Read the model definition and answer for the solid it produces. Units are mm, in the model's axes. A direction names the side the tool comes from. Coordinates: 2 decimals unless noted, no trailing zeros. Loops run counter-clockwise (first coordinate to the right, second up) from the corner with the lowest first, then second, coordinate; pieces in that order, holes last. Notation, with made-up numbers: M 80,82 L 131,82 A25 ccw 131,107 Z; hole C 24,-34 d4. An arc over 180 degrees is marked long. One line per item, written item: value. Start each with the question number.
1. Consider probe 1 along Y at (x, z) = (0, 4.15); probe 2 along X at (y, z) = (-7, 1.5); probe 3 along Y at (x, z) = (-2, -1.5). Determine where each line is inside the solid, lowest interval first.
2. For faces 4 (the face through (9, 6, 1.118)), 5 (the face through (-3.26, -14.68, -1.39)), 6 (the face through (10, -10, -2.134)), 7 (the face through (-3, -8, 3.734)), determine the directions among +Z, -Z, +X, -X, +Y, -Y from which every point of the face is accessible in a straight line to the end or side of a thin tool.
3. Determine the mould class of faces 1 (the face through (10, -10, 2.134)), 2 (the face through (8.89, 2.8, -3.29)), 3 (the face through (-8.03, 0.35, 4.07)) for opening direction X: +X half, -X half, draft (parallel to the pull), parting line (faces both ways), or undercut.
4. Flat-ended cylindrical pins translate along their axes: pin 1 (10.5 mm diameter, centred on x = 0, y = 0, fed in from -Z); pin 2 (1.5 mm diameter, centred on y = 10.5, z = 0.5, fed in from +X); pin 3 (2 mm diameter, centred on x = 0, y = -12, fed in from +Z); pin 4 (1.5 mm diameter, centred on x = 2, z = -0.5, fed in from -Y). Find the tip coordinate at first contact, or state that the pin passes through.
5. The part is cut by section A-A (z = -3.25). Write down the section's boundary in (x, y), then the cut area to 3 significant figures.
```python
from build123d import *
from build123d import SkipClean  # not in build123d's __all__

# Parameters (mm, degrees)
F2_R    = 0.889
F4_SIZE = 0.254
F5_R    = 1.27


with BuildPart() as f1:
    # F0 (on Front) → F1 (revolve)
    with BuildSketch(Plane.XZ):
        Polygon((8.0391, 2.7178), (8.0391, 0), (15.0368, 0), (15.0368, 2.1336), (13.8207983748, 2.1336), (12.3698, 1.1176), (9.3218, 1.1176), (9.3218, 4.4196), (8.0391, 4.4196), (8.0391, 3.7338), (8.8011, 3.7338), (8.8011, 2.7178), align=None)
    revolve(axis=Axis((0, 0, 18.0261821733), (0, 0, 1)))

    # F2 (on Front) → F3 (revolve, cut)
    with BuildSketch(Plane.XZ):
        with Locations((15.0368, 0)):
            Circle(F2_R)
    revolve(axis=Axis((0, 0, 18.0261821733), (0, 0, 1)), mode=Mode.SUBTRACT)

    # F4
    f4_edges = [f1.edges().sort_by_distance(p)[0] for p in [
        (-15.0368, 0, 2.1336),
        (-9.3218, 0, 4.4196),
    ]]
    chamfer(f4_edges, length=F4_SIZE)

    # F5
    f5_edges = [f1.edges().sort_by_distance(p)[0] for p in [
        (-9.3218, 0, 1.1176),
    ]]
    fillet(f5_edges, radius=F5_R)

    # F6: F1 across plane


with BuildPart() as f1_1:
    add(f1.part, clean=False)
    with SkipClean():  # cleaning this boolean's faces spoils the solid; the shape is the same uncleaned
        add(f1.part.mirror(Plane.XY), clean=False)


solid = f1_1.part
```
Answer block:
1. probe 1: y = -9.32 to -8.04, 8.04 to 9.32
1. probe 2: x = -13.31 to -10.85, -6.69 to -3.95, 3.95 to 6.69, 10.85 to 13.31
1. probe 3: y = -14.9 to -12.76, -9.47 to -7.79, 7.79 to 9.47, 12.76 to 14.9
2. face 4: +Z
2. face 5: +Z, -Z
2. face 6: -Z
2. face 7: none
3. face 1: draft
3. face 2: parting line
3. face 3: undercut
4. pin 1: passes through
4. pin 2: stops at x = 11.35
4. pin 3: stops at z = 1.56
4. pin 4: stops at y = -14.98
5. outline: C 0,0 d18.64; hole C 0,0 d17.6
5. area: 29.6 mm2
